The model under review builds one solid part; all positions refer to its coordinate system, in mm. Face numbers are marked on the shaded views. Coordinates: 2 decimals unless noted, no trailing zeros. Loops run counter-clockwise (first coordinate to the right, second up) from the corner with the lowest first, then second, coordinate; pieces in that order, holes last. Notation, with made-up numbers: (13, -17.75) - (47, -17.75) arc R23 cw to (47, -3.75) - close; hole circle Ø8 at (10, 2). An arc over 180 degrees is marked (long way). Use a Markdown table: item, result. Add a question column.
1) The part is to be moulded in two halves that separate along Z. For the marked faces 1, 2, 3 and 4, say which applies: pulls with the +Z half, pulls with the -Z half, needs draft (parallel to the pull), parting line crosses it, or undercut.
2) Add section C-C, the plane y = 90. Give the boundary of the cut face in (x, z), and give its area (3 significant figures).
3) Add section B-B, the plane y = 50. Give the boundary of the cut face in (x, z).
4) To check wall thickness, follow L1, parallel to Y at x = 2.5, z = 10; L2, parallel to Y at x = 2.25, z = 48; L3, parallel to Z at x = 2.75, y = 50. State the ranges of each line that lie inside material, in increasing order. Write a range as [from, to].
5) Add section D-D, the plane z = 10. Give the boundary of the cut face in (x, y).
6) Add section A-A, the plane z = 36. Give the boundary of the cut face in (x, y).
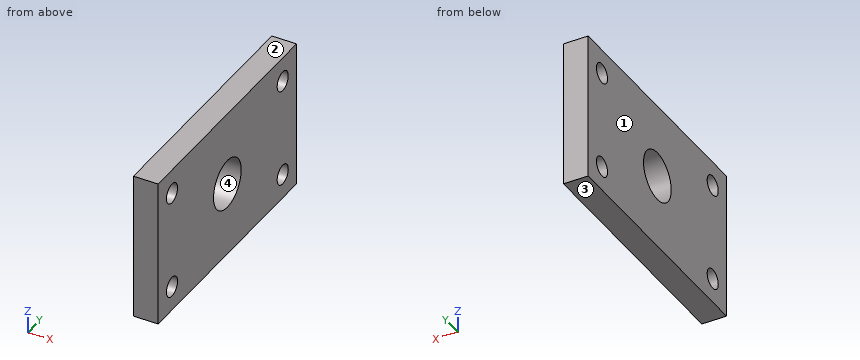
```python
from build123d import *

# Parameters (mm, degrees)
SKETCH1_W           = 100
SKETCH1_H           = 60
BOSS_EXTRUDE1_DEPTH = 10
SKETCH2_R           = 4
CUT_EXTRUDE2_DEPTH  = 118.046999107
SKETCH3_R           = 10
CUT_EXTRUDE4_DEPTH  = 118.046999107


with BuildPart() as part:
    # Sketch1 → Boss-Extrude1 (new body)
    with BuildSketch(Plane.YZ):
        with Locations((50, 30)):
            Rectangle(SKETCH1_W, SKETCH1_H)
    extrude(amount=BOSS_EXTRUDE1_DEPTH)

    # Sketch2 → Cut-Extrude2 (cut, through all)
    with BuildSketch(Plane.YZ):
        with Locations(Location((10, 10, 0), (0, 0, 270))):
            Circle(SKETCH2_R)
        with Locations(Location((90, 10, 0), (0, 0, 270))):
            Circle(SKETCH2_R)
        with Locations(Location((10, 50, 0), (0, 0, 270))):
            Circle(SKETCH2_R)
        with Locations(Location((90, 50, 0), (0, 0, 270))):
            Circle(SKETCH2_R)
    extrude(amount=CUT_EXTRUDE2_DEPTH, mode=Mode.SUBTRACT)

    # Sketch3 → Cut-Extrude4 (cut, through all)
    with BuildSketch(Plane.YZ):
        with Locations(Location((50, 30, 0), (0, 0, 270))):
            Circle(SKETCH3_R)
    extrude(amount=CUT_EXTRUDE4_DEPTH, mode=Mode.SUBTRACT)


solid = part.part
```
From the geometry:
| question | item | result |
|---|---|---|
| 1 | face 1 | needs draft |
| 1 | face 2 | pulls with the +Z half |
| 1 | face 3 | pulls with the -Z half |
| 1 | face 4 | undercut |
| 2 | outline | (0, 0) - (10, 0) - (10, 6) - (0, 6) - close; (0, 14) - (10, 14) - (10, 46) - (0, 46) - close; (0, 54) - (10, 54) - (10, 60) - (0, 60) - close |
| 2 | area | 440 mm^2 |
| 3 | outline | (0, 0) - (10, 0) - (10, 20) - (0, 20) - close; (0, 40) - (10, 40) - (10, 60) - (0, 60) - close |
| 4 | L1 | y = [0, 6], [14, 86], [94, 100] |
| 4 | L2 | y = [0, 6.54], [13.46, 86.54], [93.46, 100] |
| 4 | L3 | z = [0, 20], [40, 60] |
| 5 | outline | (0, 0) - (10, 0) - (10, 6) - (0, 6) - close; (0, 14) - (10, 14) - (10, 86) - (0, 86) - close; (0, 94) - (10, 94) - (10, 100) - (0, 100) - close |
| 6 | outline | (0, 0) - (10, 0) - (10, 42) - (0, 42) - close; (0, 58) - (10, 58) - (10, 100) - (0, 100) - close |
